```python
from build123d import *

# Parameters (mm, degrees)
BOSS_EXTRUDE7_DEPTH = 1.68
BOSS_EXTRUDE8_DEPTH = 6.695435


with BuildPart() as part:
    # Sketch23 → Boss-Extrude7 (new body)
    with BuildSketch(Plane(origin=(0, 12.527717687, 0), x_dir=(1, 0, 0), z_dir=(0, 1, 0))):
        with BuildLine():
            Line((17.863123843, 63.129446847), (14.718163043, 45.293487391))
            Line((14.718163043, 45.293487391), (34.414318061, 41.820523845))
            Line((34.414318061, 41.820523845), (37.008919102, 56.535237557))
            add(Edge.make_bspline(
                [(37.008919102, 56.535237557), (27.963542945, 60.982758463), (17.863123843, 63.129446847)],
                knots=[4.196334531, 4.196334531, 4.196334531, 4.471902655, 4.471902655, 4.471902655], degree=2, weights=[1, 0.990522784, 1]))
        make_face()
    extrude(amount=-BOSS_EXTRUDE7_DEPTH)

    # Sketch24 → Boss-Extrude8 (add)
    with BuildSketch(Plane.XZ.offset(-10.847717687)):
        with BuildLine():
            Line((16.906130039, -57.702065086), (33.647861841, -54.750046066))
            Line((33.647861841, -54.750046066), (31.459894802, -42.341468378))
            Line((31.459894802, -42.341468378), (34.414318061, -41.820523845))
            Line((34.414318061, -41.820523845), (37.008919102, -56.535237557))
            add(Edge.make_bspline(
                [(17.863123843, -63.129446847), (27.963542945, -60.982758463), (37.008919102, -56.535237557)],
                knots=[1.811282652, 1.811282652, 1.811282652, 2.086850776, 2.086850776, 2.086850776], degree=2, weights=[1, 0.990522784, 1]))
            Line((17.863123843, -63.129446847), (16.906130039, -57.702065086))
        make_face()
    extrude(amount=BOSS_EXTRUDE8_DEPTH)


solid = part.part
```
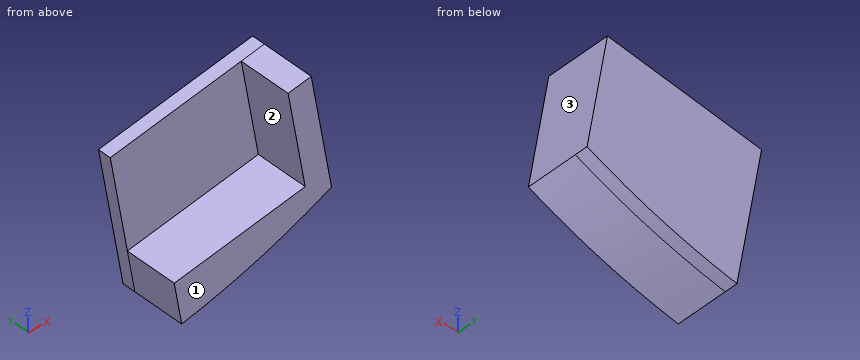
Model file for the job. Use its own axes, mm. Face numbers are marked on the shaded views. Round coordinates to 2 decimals unless told otherwise and drop trailing zeros. Order: outer loops, then holes, each group sorted by start corner. A loop starts at its lowest first (then second) coordinate and runs counter-clockwise, first axis right, second up. Notation, with made-up numbers: (-27.5, 84) -> (-5.5, 84) arc R35 cw to (-5.5, 118) -> close; hole circle Ø10 at (38.25, -21.5). An arc over 180 degrees is marked (long way). Use one line per item in the form item = value.
Item 1: Pull direction Z, two halves, no side cores. Call the marked faces 1, 2 and 3: released by +Z, released by -Z, zero draft, split by the parting line, or undercut.
Returned:
face_1 = zero draft
face_2 = undercut
face_3 = released by +Z
Item 2: Cut at B-B, the plane z = -50. Write the cut outline in (x, y), and give its area (3 significant figures).
Returned:
outline = (15.55, 10.85) -> (32.81, 10.85) -> (32.81, 4.15) -> (35.86, 4.15) -> (35.86, 12.53) -> (15.55, 12.53) -> close
area = 54.5 mm^2
Item 3: Drill centre lines: line 1 (Y direction, x = 24.25, z = -48.25); line 2 (X direction, y = 6.25, z = -54); line 3 (Z direction, x = 29.25, y = 7.75). Where is each one in solid material? Low to high.
Returned:
line_1 = 10.85 to 12.53
line_2 = 33.52 to 36.56
line_3 = -59.85 to -55.53
Item 4: Flat gauge pins, fed straight in: pin 1 Ø3 at (x, y) = (22.5, 8) entering from -Z; pin 2 Ø1.5 at (x, y) = (25, 6) entering from -Z; pin 3 Ø4 at (x, y) = (22, 11) entering from -Z. Where does each tip first touch, or does it go through?
Returned:
pin_1 = -62.4
pin_2 = -61.51
pin_3 = -62.65
Item 5: Cut at A-A, the plane z = -45. Write the cut outline in (x, y).
Returned:
outline = (16.38, 10.85) -> (31.93, 10.85) -> (31.93, 4.15) -> (34.97, 4.15) -> (34.97, 12.53) -> (16.38, 12.53) -> close
